Check sheet for the modelled part. Datum: model origin and axes. Units: mm. Face numbers are marked on the shaded views. A direction names the side the tool comes from. Round coordinates to 2 decimals unless told otherwise and drop trailing zeros. Loops run counter-clockwise (first coordinate to the right, second up) from the corner with the lowest first, then second, coordinate; pieces in that order, holes last. Notation, with made-up numbers: (2.5, -22.5) -> (23.5, -22.5) arc R17 cw to (23.5, -7.5) -> close; hole circle Ø3 at (-39, 80). An arc over 180 degrees is marked (long way). Use one line per item in the form item = value. Start each with the question number.
(1) Material ranges on probe 1 along X at (y, z) = (5.25, 5); probe 2 along Z at (x, y) = (24, 2.5); probe 3 along X at (y, z) = (10.25, 6.25), recorded low to high. Write a range as [from, to].
(2) Go/stop test with flat-tipped pins: pin 1 (3.5 mm diameter, centred on x = 24.5, y = 7, fed in from +Z); pin 2 (1 mm diameter, centred on x = 7, y = 9, fed in from -Z); pin 3 (6 mm diameter, centred on y = 2.5, z = 15.5, fed in from -X). Record where each tip stops, or that it passes through.
(3) Sectioned sample at D-D (y = 1). Record the cut outline in (x, z) (3 decimals).
(4) Set-up check for the marked faces 4, 5 and 6: record each of +Z, -Z, +X, -X, +Y, -Y from which the full face is reachable in a straight line by a thin tool's end or side.
(5) Sectioned sample at A-A (y = 5.5). Record the cut outline in (x, z) (3 decimals).
(6) Sectioned sample at B-B (z = 8.5). Record the cut outline in (x, y), and give its area (3 significant figures).
(7) Draft check along X on the marked faces 1, 2 and 3. Enter one of: released by +X, released by -X, zero draft, split by the parting line, or undercut.
(8) Sectioned sample at C-C (x = -23.5). Record the cut outline in (y, z).
from build123d import *

# Parameters (mm, degrees)
BOSS_EXTRUDE1_DEPTH = 11
SKETCH2_R           = 3
CUT_EXTRUDE1_DEPTH  = 30
CUT_EXTRUDE2_DEPTH  = 20
FILLET1_R           = 2.36


with BuildPart() as part:
    # Sketch1 → Boss-Extrude1 (new body)
    with BuildSketch(Plane(origin=(0, 0, 0), x_dir=(1, 0, 0), z_dir=(0, 1, 0))):
        with BuildLine():
            Line((-27.916231576, -22.71939994), (27.916231576, -22.71939994))
            Line((27.916231576, -22.71939994), (27.916231576, -3.602655093))
            Line((27.916231576, -3.602655093), (13.916231576, -3.602655093))
            ThreePointArc((13.916231576, -3.602655093), (0, -14.375), (-13.916231576, -3.602655093))
            Line((-13.916231576, -3.602655093), (-27.916231576, -3.602655093))
            Line((-27.916231576, -3.602655093), (-27.916231576, -22.71939994))
        make_face()
    extrude(amount=BOSS_EXTRUDE1_DEPTH)

    # Sketch2 → Cut-Extrude1 (cut)
    with BuildSketch(Plane(origin=(0, 0, 3.602655093), x_dir=(-1, 0, 0), z_dir=(0, 0, -1))):
        with Locations((21.916231576, 5.5)):
            Circle(SKETCH2_R)
        with Locations((-21.916231576, 5.5)):
            Circle(SKETCH2_R)
    extrude(amount=-CUT_EXTRUDE1_DEPTH, mode=Mode.SUBTRACT)

    # Sketch4 → Cut-Extrude2 (cut)
    with BuildSketch(Plane.XZ):
        with BuildLine():
            Line((27.916231576, 6.852655093), (27.916231576, 7.602655093))
            Line((27.916231576, 7.602655093), (27.916231576, 22.71939994))
            Line((27.916231576, 22.71939994), (-27.916231576, 22.71939994))
            Line((-27.916231576, 22.71939994), (-27.916231576, 7.602655093))
            Line((-27.916231576, 7.602655093), (-27.916231576, 6.852655093))
            Line((-27.916231576, 6.852655093), (-16.238280179, 6.852655093))
            ThreePointArc((-16.238280179, 6.852655093), (0, 17.625), (16.238280179, 6.852655093))
            Line((16.238280179, 6.852655093), (27.916231576, 6.852655093))
        make_face()
    extrude(amount=-CUT_EXTRUDE2_DEPTH, mode=Mode.SUBTRACT)

    # Fillet1
    fillet1_edges = [part.edges().sort_by_distance(p)[0] for p in [
        (27.916231576, 0, 5.227655093),
        (27.916231576, 11, 5.227655093),
        (-27.916231576, 11, 5.227655093),
        (-27.916231576, 0, 5.227655093),
    ]]
    fillet(fillet1_edges, radius=FILLET1_R)


solid = part.part
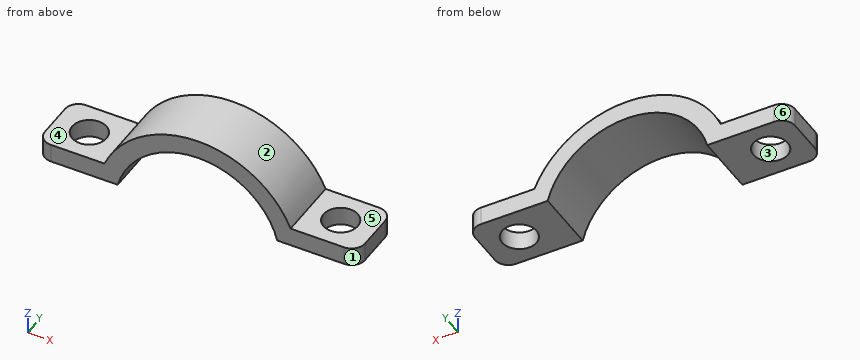
Checks:
q1.probe_1 = [-27.92, -24.91], [-18.93, -13.48], [13.48, 18.93], [24.91, 27.92]
q1.probe_2 = [3.6, 6.85]
q1.probe_3 = [-27.28, -12.95], [12.95, 27.28]
q2.pin_1 = 6.85
q2.pin_2 = 12.26
q2.pin_3 = -12.43
q3.outline = (-27.485, 3.603) -> (-13.916, 3.603) arc R14.375 cw to (13.916, 3.603) -> (27.485, 3.603) -> (27.485, 6.853) -> (16.238, 6.853) arc R17.625 ccw to (-16.238, 6.853) -> (-27.485, 6.853) -> close
q4.face_4 = +Z, -X, +Y, -Y
q4.face_5 = +Z, +X, +Y, -Y
q4.face_6 = +Z, -Z, -X, +Y
q5.outline = (-27.916, 3.603) -> (-24.916, 3.603) -> (-24.916, 6.853) -> (-27.916, 6.853) -> close; (-18.916, 3.603) -> (-13.916, 3.603) arc R14.375 cw to (13.916, 3.603) -> (18.916, 3.603) -> (18.916, 6.853) -> (16.238, 6.853) arc R17.625 ccw to (-16.238, 6.853) -> (-18.916, 6.853) -> close; (24.916, 3.603) -> (27.916, 3.603) -> (27.916, 6.853) -> (24.916, 6.853) -> close
q6.outline = (-15.44, 0) -> (-11.59, 0) -> (-11.59, 11) -> (-15.44, 11) -> close; (11.59, 0) -> (15.44, 0) -> (15.44, 11) -> (11.59, 11) -> close
q6.area = 84.6 mm2
q7.face_1 = released by +X
q7.face_2 = split by the parting line
q7.face_3 = undercut
q8.outline = (0, 3.6) -> (2.95, 3.6) -> (2.95, 6.85) -> (0, 6.85) -> close; (8.05, 3.6) -> (11, 3.6) -> (11, 6.85) -> (8.05, 6.85) -> close
